```python
from build123d import *

# Parameters (mm, degrees)
SKETCH1_R           = 10.64
BOSS_EXTRUDE1_DEPTH = 4
SKETCH2_R           = 12.875
SKETCH2_R_2         = 10.64
BOSS_EXTRUDE2_DEPTH = 4
SKETCH3_R           = 6
SKETCH3_R_2         = 4
BOSS_EXTRUDE3_DEPTH = 10
SKETCH5_R           = 2.5
CUT_EXTRUDE1_DEPTH  = 4
SKETCH6_R           = 10.64
SKETCH6_R_2         = 6
BOSS_EXTRUDE4_DEPTH = 7
SKETCH7_R           = 5.5
CUT_EXTRUDE2_DEPTH  = 4
SKETCH8_R           = 0.5
CUT_EXTRUDE3_DEPTH  = 30.964106861


with BuildPart() as part:
    # Sketch1 → Boss-Extrude1 (new body)
    with BuildSketch(Plane(origin=(0, 0, 0), x_dir=(1, 0, 0), z_dir=(0, 1, 0))):
        with BuildLine():
            Line((-4.248633652, 12.719167115), (-19.326288783, 7.682718392))
            ThreePointArc((-19.326288783, 7.682718392), (-24.86, 0), (-19.326288783, -7.682718392))
            Line((-19.326288783, -7.682718392), (-4.248633652, -12.719167115))
            ThreePointArc((-4.248633652, -12.719167115), (0, -13.41), (4.248633652, -12.719167115))
            Line((4.248633652, -12.719167115), (19.326288783, -7.682718392))
            ThreePointArc((19.326288783, -7.682718392), (24.86, 0), (19.326288783, 7.682718392))
            Line((19.326288783, 7.682718392), (4.248633652, 12.719167115))
            ThreePointArc((4.248633652, 12.719167115), (0, 13.41), (-4.248633652, 12.719167115))
        make_face()
        with Locations(Location((0, 0, 0), (0, 0, 270))):
            Circle(SKETCH1_R, mode=Mode.SUBTRACT)
    extrude(amount=BOSS_EXTRUDE1_DEPTH)

    # Sketch2 → Boss-Extrude2 (add)
    with BuildSketch(Plane(origin=(0, 4, 0), x_dir=(1, 0, 0), z_dir=(0, 1, 0))):
        with Locations(Location((0, 0, 0), (0, 0, 270))):
            Circle(SKETCH2_R)
        with Locations(Location((0, 0, 0), (0, 0, 270))):
            Circle(SKETCH2_R_2, mode=Mode.SUBTRACT)
    extrude(amount=BOSS_EXTRUDE2_DEPTH)

    # Sketch5 → Cut-Extrude1 (cut)
    with BuildSketch(Plane(origin=(0, 0, 0), x_dir=(1, 0, 0), z_dir=(0, 1, 0))):
        with Locations(Location((-18.25, 0, 0), (0, 0, 270))):
            Circle(SKETCH5_R)
        with Locations(Location((18.25, 0, 0), (0, 0, 270))):
            Circle(SKETCH5_R)
    extrude(amount=CUT_EXTRUDE1_DEPTH, mode=Mode.SUBTRACT)



with BuildPart() as body_2:
    # Sketch3 → Boss-Extrude3 (new body)
    with BuildSketch(Plane(origin=(0, 0, 0), x_dir=(1, 0, 0), z_dir=(0, 1, 0))):
        with Locations(Location((0, 0, 0), (0, 0, 270))):
            Circle(SKETCH3_R)
        with Locations(Location((0, 0, 0), (0, 0, 270))):
            Circle(SKETCH3_R_2, mode=Mode.SUBTRACT)
    extrude(amount=BOSS_EXTRUDE3_DEPTH)


with BuildPart() as part_1:
    add(part.part)

    add(body_2.part)  # Boss-Extrude4 merges body 2
    # Sketch6 → Boss-Extrude4 (add)
    with BuildSketch(Plane(origin=(0, 0, 0), x_dir=(1, 0, 0), z_dir=(0, 1, 0))):
        with Locations(Location((0, 0, 0), (0, 0, 270))):
            Circle(SKETCH6_R)
        with Locations(Location((0, 0, 0), (0, 0, 270))):
            Circle(SKETCH6_R_2, mode=Mode.SUBTRACT)
    extrude(amount=BOSS_EXTRUDE4_DEPTH)

    # Sketch7 → Cut-Extrude2 (cut)
    with BuildSketch(Plane(origin=(0, 8, 0), x_dir=(1, 0, 0), z_dir=(0, 1, 0))):
        with Locations((-18.25, 0)):
            Circle(SKETCH7_R)
        with Locations((18.25, 0)):
            Circle(SKETCH7_R)
    extrude(amount=-CUT_EXTRUDE2_DEPTH, mode=Mode.SUBTRACT)

    # Sketch8 → Cut-Extrude3 (cut, through all)
    with BuildSketch(Plane.XY):
        with Locations(Location((0, 9, 0), (0, 0, 90))):
            Circle(SKETCH8_R)
    extrude(amount=-CUT_EXTRUDE3_DEPTH, mode=Mode.SUBTRACT)


solid = part_1.part
```
Could you check a few things on this model? Use its own coordinates, in mm. A direction names the side the tool comes from. Round coordinates to 2 decimals unless told otherwise and drop trailing zeros. Write each loop counter-clockwise with the first axis right and the second up, starting at its lowest first coordinate (ties: lowest second). Pieces come first, ordered by that corner, then holes. Notation, with made-up numbers: M 23.5,-29 L 56.5,-29 A30 cw 56.5,-1 Z; hole C 88,-37.5 d8. An arc over 180 degrees is marked long. Answer in a Markdown table with one row per item. Add a question column.
Q1. If we mould it in two halves opening along Z, with no side actions, what happens to faces 6 (the cylindrical face through (1.802, 8.479, 5.723)), 7 (the cylindrical face through (0.192, 9.462, -4.97)), 8 (the flat face through (11.682, 1.972, 10.236))? For each: +Z half, -Z half, draft (parallel to the pull), parting line (faces both ways), or undercut.
Q2. On a 3-axis mill with a long thin cutter (end or side, diameter ignored), from which of +Z, -Z, +X, -X, +Y, -Y can I reach the whole of each face in a straight line? I mean faces 1 (the cylindrical face through (0.269, 5.972, -12.872)), 2 (the cylindrical face through (-0.269, 5.972, 12.872)), 3 (the cylindrical face through (12.75, 6.03, -0.01)), 4 (the cylindrical face through (-12.75, 6.03, 0.01)), 5 (the flat face through (-5, 7, 5)). Say none if no direction works.
Q3. Imagine slicing it at A-A (x = 0). Please give me the cut outline in (y, z) (3 decimals), then the cut area to 3 significant figures.
Q4. Imagine slicing it at D-D (x = 18.25). Please give me the cut outline in (y, z), then the cut area to 3 significant figures.
Q5. Imagine slicing it at C-C (y = 5.75). Please give me the cut outline in (x, z) (3 decimals).
Q6. Imagine slicing it at B-B (z = 0). Please give me the cut outline in (x, y), then the cut area to 3 significant figures.
Q7. If I drill on line 1 (X direction, y = 2.5, z = 1.5); line 2 (Z direction, x = 0, y = 2.75); line 3 (Y direction, x = 0, z = 12), over which ranges is the centre line in solid material (lowest first)? Write a range as from..to.
Q8. Will these pins go through, and if not, where does the flat tip stop? pin 1 Ø1 at (y, z) = (7, 2.5) entering from +X; pin 2 Ø5 at (y, z) = (2, 4.5) entering from -X; pin 3 Ø2 at (x, y) = (-9, 7.5) entering from -Z.
Values:
| question | item | result |
|---|---|---|
| 1 | face 6 | undercut |
| 1 | face 7 | draft |
| 1 | face 8 | +Z half |
| 2 | face 1 | -Z, +Y |
| 2 | face 2 | +Z, +Y |
| 2 | face 3 | +X, +Y |
| 2 | face 4 | -X, +Y |
| 2 | face 5 | +Y |
| 3 | outline | M 0,-13.41 L 4,-13.41 L 4,-12.875 L 8,-12.875 L 8,-10.64 L 7,-10.64 L 7,-6 L 8.5,-6 L 8.5,-4 L 0,-4 Z; M 0,4 L 10,4 L 10,6 L 7,6 L 7,10.64 L 8,10.64 L 8,12.875 L 4,12.875 L 4,13.41 L 0,13.41 Z; M 9.5,-6 L 10,-6 L 10,-4 L 9.5,-4 Z |
| 3 | area | 143 mm^2 |
| 4 | outline | M 0,-8.04 L 4,-8.04 L 4,-2.5 L 0,-2.5 Z; M 0,2.5 L 4,2.5 L 4,8.04 L 0,8.04 Z |
| 4 | area | 44.3 mm^2 |
| 5 | outline | M -12.838,-0.979 A12.875 ccw 12.838,-0.979 A5.5 cw 12.838,0.979 A12.875 ccw -12.838,0.979 A5.5 cw Z; hole C 0,0 d8 |
| 6 | outline | M -24.86,0 L -20.75,0 L -20.75,4 L -24.86,4 Z; M -15.75,0 L -4,0 L -4,10 L -6,10 L -6,7 L -10.64,7 L -10.64,8 L -12.75,8 L -12.75,4 L -15.75,4 Z; M 4,0 L 15.75,0 L 15.75,4 L 12.75,4 L 12.75,8 L 10.64,8 L 10.64,7 L 6,7 L 6,10 L 4,10 Z; M 20.75,0 L 24.86,0 L 24.86,4 L 20.75,4 Z |
| 6 | area | 196 mm^2 |
| 7 | line 1 | -24.72..-20.25, -16.25..-3.71, 3.71..16.25, 20.25..24.72 |
| 7 | line 2 | -13.41..-4, 4..13.41 |
| 7 | line 3 | 0..8 |
| 8 | pin 1 | x = 12.72 |
| 8 | pin 2 | x = -24.61 |
| 8 | pin 3 | z = -10.09 |
